The listing builds one solid part. Answer for the finished solid, in the listing's coordinates (mm). A direction names the side the tool comes from. Coordinates: 2 decimals unless noted, no trailing zeros. Loops run counter-clockwise (first coordinate to the right, second up) from the corner with the lowest first, then second, coordinate; pieces in that order, holes last. Notation, with made-up numbers: (73, -22) - (114, -22) arc R19 ccw to (114, 7) - close; hole circle Ø8 at (62.25, 33.5). An arc over 180 degrees is marked (long way). Put each result on its own line as item: value.
```python
from build123d import *

# Parameters (mm, degrees)
F1_DEPTH = 63.5
F2_DEPTH = 25.4
F3_DEPTH = 7.9375
F0_W     = 25.4
F0_H     = 19.05
F5_R     = 6.35


with BuildPart() as f1:
    # F0 (on Front) → F1 (new body, symmetric)
    with BuildSketch(Plane.XZ):
        Polygon((-41.275, 9.525), (-41.275, -9.525), (41.275, -9.525), (41.275, 9.525), (22.225, 9.525), align=None)
    extrude(amount=F1_DEPTH, both=True)

    # F0 (on Front) → F2 (join, symmetric)
    with BuildSketch(Plane.XZ):
        with BuildLine():
            Line((22.225, 9.525), (41.275, 9.525))
            Line((41.275, 9.525), (41.275, 27.0002))
            ThreePointArc((41.275, 27.0002), (45.9246798487, 38.2255201513), (57.15, 42.8752))
            Line((57.15, 42.8752), (60.325, 42.8752))
            Line((60.325, 42.8752), (60.325, 61.9252))
            Line((60.325, 61.9252), (57.15, 61.9252))
            ThreePointArc((57.15, 61.9252), (32.4542956671, 51.6959043329), (22.225, 27.0002))
            Line((22.225, 27.0002), (22.225, 9.525))
        make_face()
    extrude(amount=F2_DEPTH, both=True)

    # F0 (on Front) → F3 (join, symmetric)
    with BuildSketch(Plane.XZ):
        with BuildLine():
            add(Edge.make_bspline(
                [(-41.275, 9.525), (-41.275, 35.2953113616), (0, 61.9252), (57.15, 61.9252)],
                knots=[0, 0, 0, 0, 111.5045361635, 111.5045361635, 111.5045361635, 111.5045361635], degree=3))
            Line((-41.275, 9.525), (22.225, 9.525))
            Line((22.225, 9.525), (22.225, 27.0002))
            ThreePointArc((22.225, 27.0002), (32.4542956671, 51.6959043329), (57.15, 61.9252))
        make_face()
    extrude(amount=F3_DEPTH, both=True)

    # F0 (on Front) → F4 (revolve)
    with BuildSketch(Plane.XZ):
        with Locations((73.025, 52.4002)):
            Rectangle(F0_W, F0_H)
    revolve(axis=Axis((60.325, 0, 52.3875), (0, 0, -1)))

    # F5
    f5_edges = [f1.edges().sort_by_distance(p)[0] for p in [
        (-41.275, -63.5, 0),
        (41.275, -63.5, 0),
        (41.275, 63.5, 0),
        (-41.275, 63.5, 0),
    ]]
    fillet(f5_edges, radius=F5_R)


solid = f1.part
```
1) Straight lines are drawn through the part: L1, parallel to Z at x = 0, y = -8 (3 decimals); L2, parallel to Y at x = -18.5, z = 35; L3, parallel to Y at x = 36, z = 46.5. For each, find the intervals that lie inside material, in ascending order. Write a range as [from, to].
Found:
L1: z = [-9.525, 9.525]
L2: y = [-7.94, 7.94]
L3: y = [-25.4, 25.4]
2) Each of these flat-tipped pins is pushed along its axis until it touches: pin 1 (1 mm diameter, centred on x = 60.5, z = 49, fed in from +Y); pin 2 (19 mm diameter, centred on y = -18.5, z = 22, fed in from -X) (3 decimals); pin 3 (8 mm diameter, centred on x = 34, y = 37, fed in from +Z) (3 decimals). Where does it stop, or does it pass through?
Found:
pin 1: stops at y = 25.4
pin 2: stops at x = 22.225
pin 3: stops at z = 9.525
3) The part is cut by section B-B (x = 53.5). Give the vertices of the cut face in (y, z).
Found:
outline: (-25.4, 42.45) - (25.4, 42.45) - (25.4, 61.73) - (24.47, 61.73) - (24.47, 61.93) - (-24.47, 61.93) - (-24.47, 61.73) - (-25.4, 61.73) - close
4) For faces 4 (the face through (0, 63.5, 0)), 5 (the face through (41.275, -1, 4)), 6 (the face through (28.763, -16.791, 47.346)), 7 (the face through (37, 25.4, 36)), 8 (the face through (22.225, 17, 18)), determine the directions among +Z, -Z, +X, -X, +Y, -Y from which every point of the face is accessible in a straight line to the end or side of a thin tool.
Found:
face 4: +Z, -Z, +X, -X, +Y
face 5: -Z, +X, +Y, -Y
face 6: +Z, -X, -Y
face 7: +Z, +X, -X, +Y
face 8: +Z, -X, +Y
5) The part is cut by section A-A (y = 51.5). Give the vertices of the cut face in (x, z) (3 decimals).
Found:
outline: (-41.275, -9.525) - (41.275, -9.525) - (41.275, 9.525) - (-41.275, 9.525) - close
6) For a pull along Y with two mould halves and no side action, classify faces 1 (the face through (1, -36, 9.525)), 2 (the face through (0, -63.5, 0)), 3 (the face through (-2, 7.938, 30)) as pulls with the +Y half, pulls with the -Y half, needs draft (parallel to the pull), parting line crosses it, or undercut.
Found:
face 1: needs draft
face 2: pulls with the -Y half
face 3: pulls with the +Y half
